```python
from build123d import *

# Parameters (mm, degrees)
SKETCH1_W           = 120
SKETCH1_H           = 90
BOSS_EXTRUDE1_DEPTH = 22.2
SHELL1_T            = -2
SKETCH2_W           = 9
SKETCH2_H           = 9
BOSS_EXTRUDE2_DEPTH = 20.2
SKETCH5_W           = 120
SKETCH5_H           = 90
SKETCH5_W_2         = 117.8
SKETCH5_H_2         = 87.8
CUT_EXTRUDE2_DEPTH  = 1
SKETCH6_R           = 2
CUT_EXTRUDE3_DEPTH  = 25
SKETCH13_R          = 3
CUT_EXTRUDE8_DEPTH  = 15
SKETCH14_W          = 50
SKETCH14_H          = 3
BOSS_EXTRUDE4_DEPTH = 10
SKETCH15_W          = 44
SKETCH15_H          = 4
CUT_EXTRUDE9_DEPTH  = 10
SKETCH16_W          = 50
SKETCH16_H          = 3
BOSS_EXTRUDE5_DEPTH = 10
SKETCH17_W          = 44
SKETCH17_H          = 4
CUT_EXTRUDE10_DEPTH = 10
SKETCH22_W          = 14.5
SKETCH22_H          = 10
SKETCH22_W_2        = 18
CUT_EXTRUDE15_DEPTH = 10
SKETCH23_W          = 10
SKETCH23_H          = 6
CUT_EXTRUDE16_DEPTH = 10
FILLET1_R           = 10
FILLET4_R           = 5
FILLET9_R           = 2
SKETCH26_R          = 3
BOSS_EXTRUDE7_DEPTH = 3
SKETCH27_R          = 1.55
CUT_EXTRUDE17_DEPTH = 2


with BuildPart() as part:
    # Sketch1 → Boss-Extrude1 (new body)
    with BuildSketch(Plane(origin=(0, 0, 0), x_dir=(1, 0, 0), z_dir=(0, 1, 0))):
        with Locations((60, 45)):
            Rectangle(SKETCH1_W, SKETCH1_H)
    extrude(amount=BOSS_EXTRUDE1_DEPTH)

    # Shell1
    shell1_openings = [part.faces().sort_by_distance(p)[0] for p in [
        (60, 22.2, -45),
    ]]
    offset(amount=SHELL1_T, openings=shell1_openings, kind=Kind.INTERSECTION)

    # Sketch2 → Boss-Extrude2 (add)
    with BuildSketch(Plane(origin=(0, 2, 0), x_dir=(1, 0, 0), z_dir=(0, 1, 0))):
        with Locations((6.5, 6.5)):
            Rectangle(SKETCH2_W, SKETCH2_H)
        with Locations((113.5, 83.5)):
            Rectangle(SKETCH2_W, SKETCH2_H)
        with Locations((113.5, 6.5)):
            Rectangle(SKETCH2_W, SKETCH2_H)
        with Locations((6.5, 83.5)):
            Rectangle(SKETCH2_W, SKETCH2_H)
    extrude(amount=BOSS_EXTRUDE2_DEPTH)

    # Sketch5 → Cut-Extrude2 (cut)
    with BuildSketch(Plane(origin=(0, 22.2, 0), x_dir=(1, 0, 0), z_dir=(0, 1, 0))):
        with Locations((60, 45)):
            Rectangle(SKETCH5_W, SKETCH5_H)
        with Locations((60, 45)):
            Rectangle(SKETCH5_W_2, SKETCH5_H_2, mode=Mode.SUBTRACT)
    extrude(amount=-CUT_EXTRUDE2_DEPTH, mode=Mode.SUBTRACT)

    # Sketch6 → Cut-Extrude3 (cut)
    with BuildSketch(Plane(origin=(0, 22.2, 0), x_dir=(1, 0, 0), z_dir=(0, 1, 0))):
        with Locations(Location((114.5, 84.5, 0), (0, 0, 270))):
            Circle(SKETCH6_R)
        with Locations(Location((114.5, 5.5, 0), (0, 0, 270))):
            Circle(SKETCH6_R)
        with Locations(Location((5.5, 84.5, 0), (0, 0, 270))):
            Circle(SKETCH6_R)
        with Locations(Location((5.5, 5.5, 0), (0, 0, 270))):
            Circle(SKETCH6_R)
    extrude(amount=-CUT_EXTRUDE3_DEPTH, mode=Mode.SUBTRACT)

    # Sketch13 → Cut-Extrude8 (cut)
    with BuildSketch(Plane.XZ):
        with Locations(Location((114.5, -5.5, 0), (0, 0, 270))):
            Circle(SKETCH13_R)
        with Locations(Location((114.5, -84.5, 0), (0, 0, 270))):
            Circle(SKETCH13_R)
        with Locations(Location((5.5, -5.5, 0), (0, 0, 270))):
            Circle(SKETCH13_R)
        with Locations(Location((5.5, -84.5, 0), (0, 0, 270))):
            Circle(SKETCH13_R)
    extrude(amount=-CUT_EXTRUDE8_DEPTH, mode=Mode.SUBTRACT)

    # Sketch14 → Boss-Extrude4 (add)
    with BuildSketch(Plane.XY):
        with Locations((70, 1.5)):
            Rectangle(SKETCH14_W, SKETCH14_H)
    extrude(amount=BOSS_EXTRUDE4_DEPTH)

    # Sketch15 → Cut-Extrude9 (cut)
    with BuildSketch(Plane(origin=(0, 0, 0), x_dir=(-1, 0, 0), z_dir=(0, -1, 0))):
        with Locations((-70, -5)):
            Rectangle(SKETCH15_W, SKETCH15_H)
    extrude(amount=-CUT_EXTRUDE9_DEPTH, mode=Mode.SUBTRACT)

    # Sketch16 → Boss-Extrude5 (add)
    with BuildSketch(Plane(origin=(0, 0, -90), x_dir=(-1, 0, 0), z_dir=(0, 0, -1))):
        with Locations((-70, 1.5)):
            Rectangle(SKETCH16_W, SKETCH16_H)
    extrude(amount=BOSS_EXTRUDE5_DEPTH)

    # Sketch17 → Cut-Extrude10 (cut)
    with BuildSketch(Plane(origin=(0, 0, 0), x_dir=(-1, 0, 0), z_dir=(0, -1, 0))):
        with Locations((-70, 95)):
            Rectangle(SKETCH17_W, SKETCH17_H)
    extrude(amount=-CUT_EXTRUDE10_DEPTH, mode=Mode.SUBTRACT)

    # Sketch22 → Cut-Extrude15 (cut)
    with BuildSketch(Plane.ZY):
        with Locations((-70.75, 12)):
            Rectangle(SKETCH22_W, SKETCH22_H)
        with Locations((-51.5, 12)):
            Rectangle(SKETCH22_W_2, SKETCH22_H)
    extrude(amount=-CUT_EXTRUDE15_DEPTH, mode=Mode.SUBTRACT)

    # Sketch23 → Cut-Extrude16 (cut)
    with BuildSketch(Plane(origin=(0, 0, -90), x_dir=(-1, 0, 0), z_dir=(0, 0, -1))):
        with Locations((-70, 11.5)):
            Rectangle(SKETCH23_W, SKETCH23_H)
    extrude(amount=-CUT_EXTRUDE16_DEPTH, mode=Mode.SUBTRACT)

    # Fillet1
    fillet1_edges = [part.edges().sort_by_distance(p)[0] for p in [
        (95, 1.5, -90),
        (95, 1.5, 0),
        (45, 1.5, 0),
        (45, 1.5, -90),
    ]]
    fillet(fillet1_edges, radius=FILLET1_R - 0.0001)  # a hair under: the kernel refuses the full size

    # Fillet4
    fillet4_edges = [part.edges().sort_by_distance(p)[0] for p in [
        (11, 12.1, -11),
        (109, 12.1, -79),
        (11, 12.1, -79),
        (109, 12.1, -11),
    ]]
    fillet(fillet4_edges, radius=FILLET4_R)

    # Fillet9
    fillet9_edges = [part.edges().sort_by_distance(p)[0] for p in [
        (0, 10.6, -90),
        (120, 10.6, -90),
        (120, 10.6, 0),
        (0, 10.6, 0),
    ]]
    fillet(fillet9_edges, radius=FILLET9_R)

    # Sketch26 → Boss-Extrude7 (add)
    with BuildSketch(Plane(origin=(0, 2, 0), x_dir=(1, 0, 0), z_dir=(0, 1, 0))):
        with Locations(Location((16.75, 83.2, 0), (0, 0, 90))):
            Circle(SKETCH26_R)
        with Locations(Location((16.75, 35, 0), (0, 0, 90))):
            Circle(SKETCH26_R)
        with Locations(Location((57.4, 35, 0), (0, 0, 90))):
            Circle(SKETCH26_R)
        with Locations(Location((57.4, 83.2, 0), (0, 0, 90))):
            Circle(SKETCH26_R)
    extrude(amount=BOSS_EXTRUDE7_DEPTH)

    # Sketch27 → Cut-Extrude17 (cut)
    with BuildSketch(Plane(origin=(0, 5, 0), x_dir=(1, 0, 0), z_dir=(0, 1, 0))):
        with Locations(Location((57.4, 83.2, 0), (0, 0, 270))):
            Circle(SKETCH27_R)
        with Locations(Location((57.4, 35, 0), (0, 0, 270))):
            Circle(SKETCH27_R)
        with Locations(Location((16.75, 35, 0), (0, 0, 270))):
            Circle(SKETCH27_R)
        with Locations(Location((16.75, 83.2, 0), (0, 0, 270))):
            Circle(SKETCH27_R)
    extrude(amount=-CUT_EXTRUDE17_DEPTH, mode=Mode.SUBTRACT)


solid = part.part
```
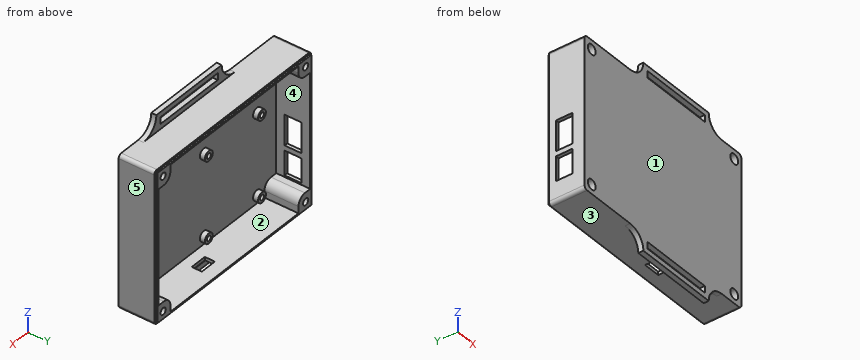
CAD build for the part. Positions are in the model's coordinates, mm. Face numbers are marked on the shaded views. A direction names the side the tool comes from. Give positions to 0.01 mm unless a question says otherwise; leave off trailing zeros. Order: outer loops, then holes, each group sorted by start corner. A loop starts at its lowest first (then second) coordinate and runs counter-clockwise, first axis right, second up. Notation, with made-up numbers: M 47,64.25 L 74,64.25 A23 ccw 74,102.25 Z; hole C 3.5,-5 d11. An arc over 180 degrees is marked long. Put each result on its own line as item: value. Start each with the question number.
(1) Saw through at D-D, the plane x = 67.5. Write the cut outline in (y, z).
(2) Drill centre lines: line 1 along X through (y, z) = (19.75, -5.5); line 2 along X through (y, z) = (15.75, -17); line 3 along X through (y, z) = (4.3, -35). Where is each one in solid material? Low to high.
(3) Saw through at A-A, the plane z = -26. Write the cut outline in (x, y), then the cut area to 3 significant figures.
(4) Saw through at B-B, the plane x = 90. Write the cut outline in (y, z).
(5) Saw through at C-C, the plane y = 10. Give the number of separate pieces and of enclosed holes in the cut face, then the cut area to 3 significant figures.
(6) Flat gauge pins, fed straight in: pin 1 Ø5 at (x, y) = (82, 16) entering from -Z; pin 2 Ø2 at (x, y) = (4.5, 14) entering from +Z; pin 3 Ø0.9 at (x, z) = (16.5, -34.5) entering from +Y. Where does each tip first touch, or does it go through?
(7) Which spindle directions (+Z, -Z, +X, -X, +Y, -Y) get a long thin tool onto all of the face, cutting with end or side? Do the marked faces 1 and 2. Say none if no direction does.
(8) Mould opens along Z. For the marked faces 3, 4 and 5 say: +Z half, -Z half, draft (parallel to the pull), parting line (faces both ways), or undercut.
Check result:
1. outline: M 0,-100 L 3,-100 L 3,-97 L 0,-97 Z; M 0,-93 L 3,-93 L 3,-90 L 8.5,-90 L 8.5,-88 L 2,-88 L 2,-2 L 22.2,-2 L 22.2,-1.1 L 21.2,-1.1 L 21.2,0 L 3,0 L 3,3 L 0,3 Z; M 0,7 L 3,7 L 3,10 L 0,10 Z; M 14.5,-90 L 21.2,-90 L 21.2,-88.9 L 22.2,-88.9 L 22.2,-88 L 14.5,-88 Z
2. line 1: x = 0 to 3.5, 7.5 to 11, 109 to 112.5, 116.5 to 120
2. line 2: x = 0 to 2, 118 to 120
2. line 3: x = 0 to 2, 13.75 to 15.2, 18.3 to 19.75, 54.4 to 55.85, 58.95 to 60.4, 118 to 120
3. outline: M 0,0 L 120,0 L 120,21.2 L 118.9,21.2 L 118.9,22.2 L 118,22.2 L 118,2 L 2,2 L 2,22.2 L 1.1,22.2 L 1.1,21.2 L 0,21.2 Z
3. area: 319 mm2
4. outline: M 0,-100 L 3,-100 L 3,-97 L 0,-97 Z; M 0,-93 L 3,-93 L 3,-90 L 21.2,-90 L 21.2,-88.9 L 22.2,-88.9 L 22.2,-88 L 2,-88 L 2,-2 L 22.2,-2 L 22.2,-1.1 L 21.2,-1.1 L 21.2,0 L 3,0 L 3,3 L 0,3 Z; M 0,7 L 3,7 L 3,10 L 0,10 Z
5. separate pieces: 3
5. enclosed holes: 4
5. area: 925 mm2
6. pin 1: stops at z = -90
6. pin 2: stops at z = 0
6. pin 3: stops at y = 3
7. face 1: +Z, -Z, +X, -X, -Y
7. face 2: +Y
8. face 3: -Z half
8. face 4: undercut
8. face 5: draft
